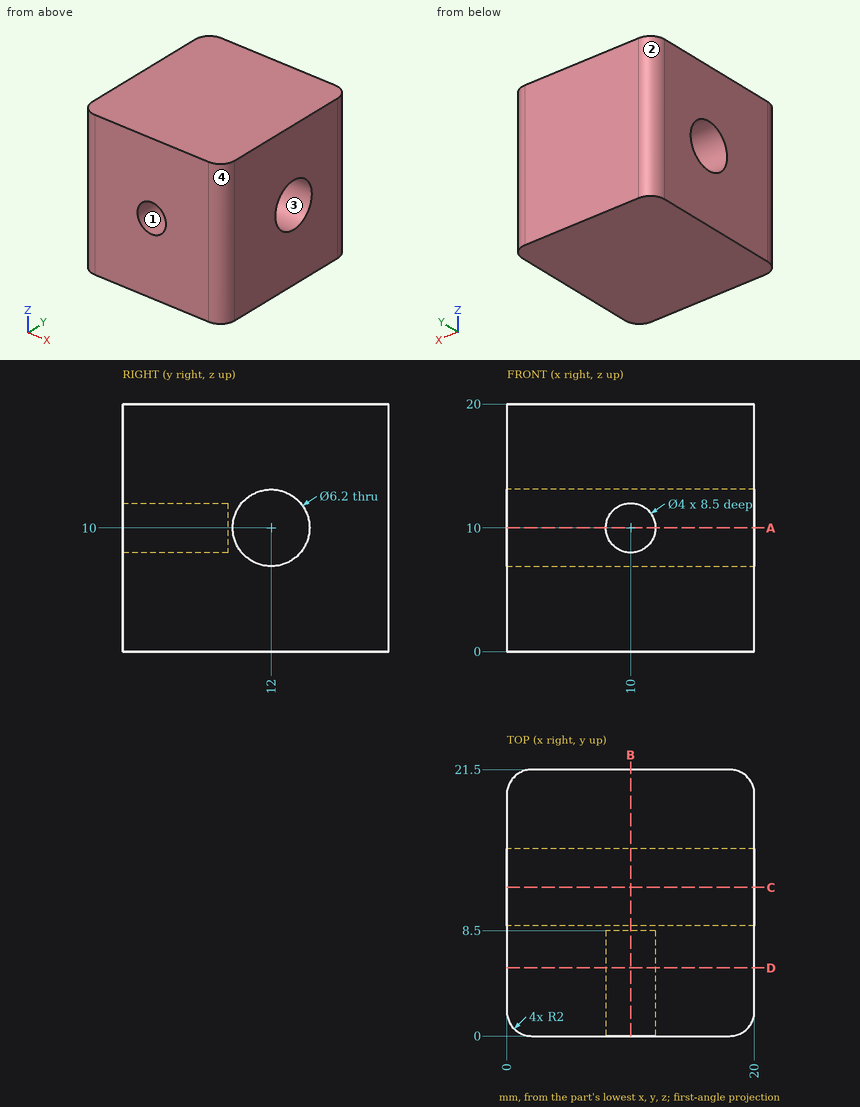
Geometry check sheet. Reference: drawing and pictorial views, mm from the part's lowest x, y, z. Round coordinates to 2 decimals unless told otherwise and drop trailing zeros. Write each loop counter-clockwise with the first axis right and the second up, starting at its lowest first coordinate (ties: lowest second). Pieces come first, ordered by that corner, then holes.
1. Section check C-C on y = 12. Enter the section's corners in (x, z).
2. Section check D-D on y = 5.5. Enter the section's corners in (x, z).
3. Draft check along Y on the marked faces 1, 2, 3 and 4. Enter one of: +Y half, -Y half, draft (parallel to the pull), parting line (faces both ways), or undercut.
4. Scan lines: L1, parallel to Z at x = 7, y = 12; L2, parallel to Y at x = 9.25, z = 10; L3, parallel to Y at x = 13, z = 10. Record each from-to range of solid material in increasing order.
5. Section check A-A on z = 10. Enter the section's corners in (x, y).
6. Section check B-B on x = 10. Enter the section's corners in (y, z).
Answer:
1. outline: (0, 0) - (20, 0) - (20, 6.9) - (0, 6.9) - close; (0, 13.1) - (20, 13.1) - (20, 20) - (0, 20) - close
2. outline: (0, 0) - (20, 0) - (20, 20) - (0, 20) - close; hole circle Ø4 at (10, 10)
3. face 1: draft
3. face 2: +Y half
3. face 3: undercut
3. face 4: -Y half
4. L1: z = 0 to 6.9, 13.1 to 20
4. L2: y = 8.5 to 8.9, 15.1 to 21.5
4. L3: y = 0 to 8.9, 15.1 to 21.5
5. outline: (0, 2) arc R2 ccw to (2, 0) - (8, 0) - (8, 8.5) - (12, 8.5) - (12, 0) - (18, 0) arc R2 ccw to (20, 2) - (20, 8.9) - (0, 8.9) - close; (0, 15.1) - (20, 15.1) - (20, 19.5) arc R2 ccw to (18, 21.5) - (2, 21.5) arc R2 ccw to (0, 19.5) - close
6. outline: (0, 0) - (21.5, 0) - (21.5, 20) - (0, 20) - (0, 12) - (8.5, 12) - (8.5, 8) - (0, 8) - close; hole circle Ø6.2 at (12, 10)
